```python
from build123d import *

# Parameters (mm, degrees)
F1_DEPTH  = 25.4
F2_R      = 6.3918462825
F3_DEPTH  = 25.401
F4_R      = 6.3541975942
F5_DEPTH  = 25.401
F6_W      = 70.0357761234
F6_H      = 27.4913627654
F7_DEPTH  = 50.8
F9_DEPTH  = 126.9250129275
F10_R     = 6.2560049958
F11_DEPTH = 126.9250129275
F13_DEPTH = 37.709375603


with BuildPart() as f1:
    # F0 (on Top) → F1 (new body)
    with BuildSketch(Plane.XY):
        with BuildLine():
            Line((75.9690925479, 21.5900018811), (-75.9690925479, 21.5900018811))
            ThreePointArc((-75.9690925479, 21.5900018811), (-97.1712359727, -1.524181319), (-76.4309093356, -25.0536352396))
            Line((-76.4309093356, -25.0536352396), (75.738184154, -25.0536352396))
            ThreePointArc((75.738184154, -25.0536352396), (96.0904147546, -1.8319984366), (75.9690925479, 21.5900018811))
        make_face()
    extrude(amount=F1_DEPTH)

    # F2 (on face) → F3 (cut, through all)
    with BuildSketch(Plane.XY.offset(25.4)):
        with Locations((-76.4309093356, 0)):
            Circle(F2_R)
    extrude(amount=-F3_DEPTH, mode=Mode.SUBTRACT)

    # F4 (on face) → F5 (cut, through all)
    with BuildSketch(Plane.XY.offset(25.4)):
        with Locations((75.9690925479, 0)):
            Circle(F4_R)
    extrude(amount=-F5_DEPTH, mode=Mode.SUBTRACT)

    # F6 (on face) → F7 (join)
    with BuildSketch(Plane.XY.offset(25.4)):
        with Locations((4.1845785454, -2.3726923391)):
            Rectangle(F6_W, F6_H)
    extrude(amount=F7_DEPTH)

    # F8 (on face) → F9 (cut, through all)
    with BuildSketch(Plane(origin=(-30.8333095163, 0, 0), x_dir=(0, -1, 0), z_dir=(-1, 0, 0))):
        with BuildLine():
            ThreePointArc((-11.3729890436, 64.7699981928), (-6.5658296023, 72.9691803573), (2.3726923391, 76.2))
            Line((2.3726923391, 76.2), (-11.3729890436, 76.2))
            Line((-11.3729890436, 76.2), (-11.3729890436, 64.7699981928))
        make_face()
        with BuildLine():
            Line((16.1183737218, 76.2), (2.3726923391, 76.2))
            ThreePointArc((2.3726923391, 76.2), (11.3112142805, 72.9691803573), (16.1183737218, 64.7699981928))
            Line((16.1183737218, 64.7699981928), (16.1183737218, 76.2))
        make_face()
    extrude(amount=-F9_DEPTH, mode=Mode.SUBTRACT)

    # F10 (on face) → F11 (cut, through all)
    with BuildSketch(Plane(origin=(-30.8333095163, 0, 0), x_dir=(0, -1, 0), z_dir=(-1, 0, 0))):
        with Locations((2.3726923391, 62.2197442057)):
            Circle(F10_R)
    extrude(amount=-F11_DEPTH, mode=Mode.SUBTRACT)

    # F12 (on face) → F13 (cut, through all)
    with BuildSketch(Plane.XZ.offset(16.1183737218)):
        Polygon((-11.6325737908, 78.8554549217), (-11.6325737908, 43.2954542339), (20.6946991384, 43.2954542339), (20.9256093949, 43.2954542339), (20.9256093949, 78.8554549217), align=None)
        with BuildLine():
            Line((20.6946991384, 43.2954542339), (-11.6325737908, 43.2954542339))
            ThreePointArc((-11.6325737908, 43.2954542339), (4.5310626738, 29.7328506966), (20.6946991384, 43.2954542339))
        make_face()
    extrude(amount=-F13_DEPTH, mode=Mode.SUBTRACT)


solid = f1.part
```
The listing builds one solid part. Answer for the finished solid, in the listing's coordinates (mm). A direction names the side the tool comes from. Give positions to 0.01 mm unless a question says otherwise; leave off trailing zeros. Order: outer loops, then holes, each group sorted by start corner. A loop starts at its lowest first (then second) coordinate and runs counter-clockwise, first axis right, second up. Notation, with made-up numbers: (46.5, 11) -> (72.5, 11) arc R25 cw to (72.5, 45) -> close; hole circle Ø1 at (40.5, -16.75). An arc over 180 degrees is marked (long way). One line per item, written item: value.
1) Flat-ended cylindrical pins translate along their axes: P1, Ø10, axis at x = -76.43, y = 0, coming from the -Z side; P2, Ø23.5, axis at x = -41, y = 5.5, coming from the +Z side; P3, Ø5, axis at x = -40.5, y = 7.5, coming from the +Z side; P4, Ø20, axis at y = -2.37, z = 62.22, coming from the +X side. Find the tip coordinate at first contact, or state that the pin passes through.
Reported:
P1: passes through
P2: stops at z = 76.06
P3: stops at z = 25.4
P4: stops at x = 39.2
2) Determine the mould class of faces 1 (the flat face through (-2, -1, 0)), 2 (the cylindrical face through (-97.16, -1.04, 12.52)), 3 (the flat face through (1, 21.59, 13)), 4 (the cylindrical face through (29.936, -1.558, 68.423)) for opening direction Y: pulls with the +Y half, pulls with the -Y half, needs draft (parallel to the pull), parting line crosses it, or undercut.
Reported:
face 1: needs draft
face 2: parting line crosses it
face 3: pulls with the +Y half
face 4: undercut
3) Find section B-B, the plane y = 0. Count the separate pieces of the cut face and the enclosed holes in it, plus the area to 3 significant figures.
Reported:
separate pieces: 5
enclosed holes: 0
area: 5,970 mm^2
4) Find section D-D, the plane x = -63.5. Determine the outline of the cut face in (y, z).
Reported:
outline: (-25.05, 0) -> (21.59, 0) -> (21.59, 25.4) -> (-25.05, 25.4) -> close
5) Find section A-A, the plane z = 52.5. Determine the outline of the cut face in (x, y), plus the area to 3 significant figures.
Reported:
outline: (-30.83, -16.12) -> (-11.63, -16.12) -> (-11.63, 11.37) -> (-30.83, 11.37) -> close; (20.93, -16.12) -> (39.2, -16.12) -> (39.2, 11.37) -> (20.93, 11.37) -> close
area: 1,030 mm^2
6) Find section C-C, the plane z = 11.5. Determine the outline of the cut face in (x, y), plus the area to 3 significant figures.
Reported:
outline: (-76.43, -25.05) -> (75.74, -25.05) arc R23.56 ccw to (75.97, 21.59) -> (-75.97, 21.59) arc R23.45 ccw to start; hole circle Ø12.78 at (-76.43, 0); hole circle Ø12.71 at (75.97, 0)
area: 8,300 mm^2
7) Find the intervals of material crossed by line 1 (Y direction, x = 29, z = 62.5); line 2 (Z direction, x = -56.5, y = 19); line 3 (Y direction, x = 32, z = 26.5), in increasing order.
Reported:
line 1: y = -16.12 to -8.62, 3.88 to 11.37
line 2: z = 0 to 25.4
line 3: y = -16.12 to 11.37
8) A tool of negligible diameter and unlimited length cuts with its end or side. For faces 5 (the flat face through (20.926, -6, 56)), 6 (the flat face through (-4.1, -16.118, 31.7)), 7 (the flat face through (39.202, -3, 50)), 8 (the flat face through (-30.833, -3, 50)), from which of +Z, -Z, +X, -X, +Y, -Y can it reach the whole face along a straight path? Write none if from no direction.
Reported:
face 5: +Z, +Y, -Y
face 6: +Z, +X, -X, -Y
face 7: +Z, +X, +Y, -Y
face 8: +Z, -X, +Y, -Y
